The figure shows three views and two pictorial views of one solid part (mm, origin at its lowest corner). Answer the questions. A direction names the side the tool comes from. Round coordinates to 2 decimals unless told otherwise and drop trailing zeros. Order: outer loops, then holes, each group sorted by start corner. A loop starts at its lowest first (then second) coordinate and runs counter-clockwise, first axis right, second up. Notation, with made-up numbers: (-38.75, -34.75) - (-11.75, -34.75) arc R33 ccw to (-11.75, -3.75) - close; hole circle Ø1 at (-10, 61). An arc over 180 degrees is marked (long way). One line per question, with ' | ' between items. Start each with the question number.
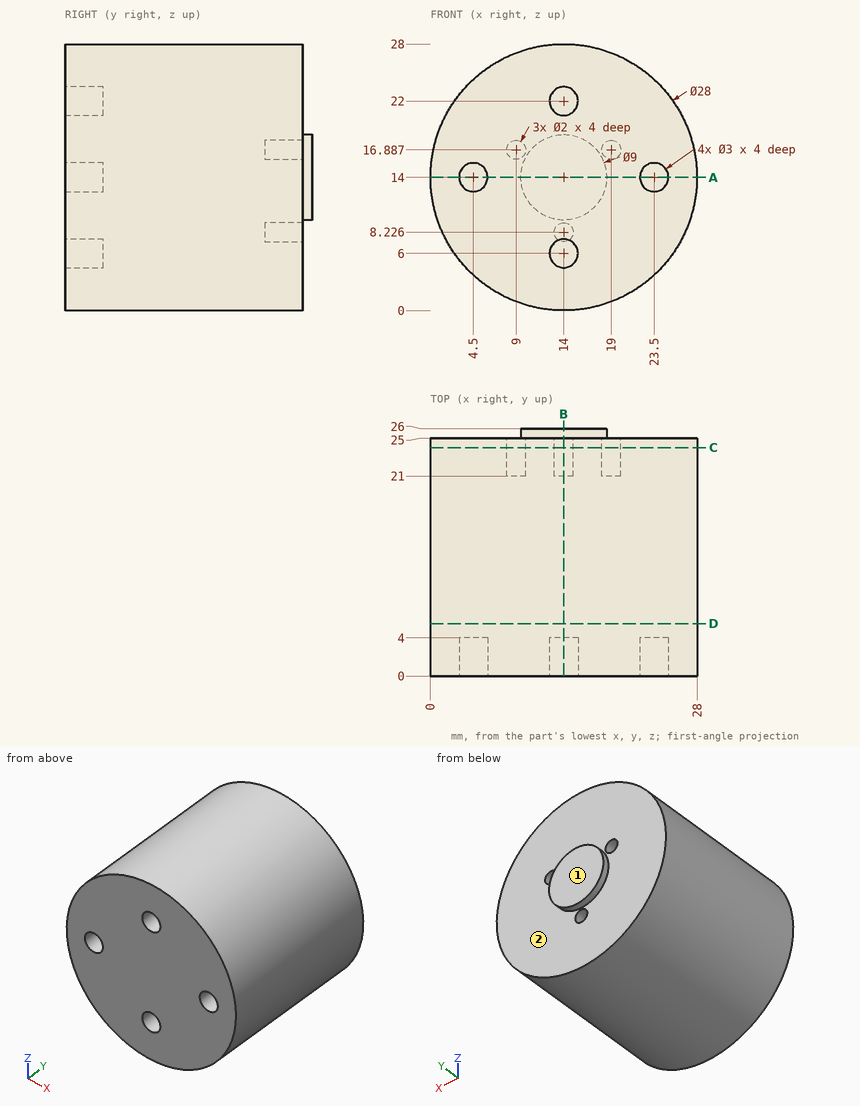
1) Section B-B on x = 14 is taken. Give the vertices of the cut face in (y, z).
2) Straight lines are drawn through the part: line 1 (X direction, y = 2.25, z = 14); line 2 (Z direction, x = 13.5, y = 10.5); line 3 (X direction, y = 23, z = 17) (1 decimal). For each, find the intervals that lie inside material, in ascending order.
3) Section C-C on y = 24 is taken. Give the vertices of the cut face in (x, z), and give its area (3 significant figures).
4) Flat-ended cylindrical pins translate along their axes: pin 1 (2.5 mm diameter, centred on x = 23.5, z = 14, fed in from +Y); pin 2 (1.5 mm diameter, centred on y = 13.5, z = 23.5, fed in from +X); pin 3 (3 mm diameter, centred on x = 7, y = 15, fed in from +Z) (1 decimal). Find the tip coordinate at first contact, or state that the pin passes through.
5) Section A-A on z = 14 is taken. Give the vertices of the cut face in (x, y).
6) For the marked faces 1 and 2, determine the directions among +Z, -Z, +X, -X, +Y, -Y from which every point of the face is accessible in a straight line to the end or side of a thin tool.
7) Section D-D on y = 5.5 is taken. Give the vertices of the cut face in (x, z), and give its area (3 significant figures).
Recorded:
1) outline: (0, 0) - (25, 0) - (25, 7.23) - (21, 7.23) - (21, 9.23) - (25, 9.23) - (25, 9.5) - (26, 9.5) - (26, 18.5) - (25, 18.5) - (25, 28) - (0, 28) - (0, 23.5) - (4, 23.5) - (4, 20.5) - (0, 20.5) - (0, 7.5) - (4, 7.5) - (4, 4.5) - (0, 4.5) - close
2) line 1: x = 0 to 3, 6 to 22, 25 to 28 | line 2: z = 0.01 to 27.99 | line 3: x = 0.3 to 8, 10 to 18, 20 to 27.7
3) outline: circle Ø28 at (14, 14); hole circle Ø2 at (9, 16.89); hole circle Ø2 at (14, 8.23); hole circle Ø2 at (19, 16.89) | area: 606 mm²
4) pin 1: stops at y = 25 | pin 2: stops at x = 24.93 | pin 3: stops at z = 26.9
5) outline: (0, 0) - (3, 0) - (3, 4) - (6, 4) - (6, 0) - (22, 0) - (22, 4) - (25, 4) - (25, 0) - (28, 0) - (28, 25) - (18.5, 25) - (18.5, 26) - (9.5, 26) - (9.5, 25) - (0, 25) - close
6) face 1: +Z, -Z, +X, -X, +Y | face 2: +Y
7) outline: circle Ø28 at (14, 14) | area: 616 mm²
